Can you work these out from the model? Positions are in its coordinate system, mm. A direction names the side the tool comes from. Round coordinates to 2 decimals unless told otherwise and drop trailing zeros. Loops run counter-clockwise (first coordinate to the right, second up) from the corner with the lowest first, then second, coordinate; pieces in that order, holes last. Notation, with made-up numbers: (-39.75, 86) -> (-32.75, 86) arc R21 ccw to (-32.75, 117) -> close; hole circle Ø5 at (-37.75, 57.25). An arc over 180 degrees is marked (long way). Use a Markdown table: item, result.
Autodesk Inventor part; units mm, degrees
ref_plane "YZ Plane" through (0, 0, 0) normal (1, 0, 0) x (0, 1, 0)
ref_plane "XZ Plane" through (0, 0, 0) normal (0, 1, 0) x (-1, 0, 0)
ref_plane "XY Plane" through (0, 0, 0) normal (0, 0, 1) x (1, 0, 0)
sketch "Sketch1" plane through (0, 0, 0) normal (0, 1, 0) x (-1, 0, 0)
  arc A0 (23.1118, 83.4134) -> (26.1118, 83.4134) centre (24.6118, 83.4134) ccw
  line L0 (23.1118, 98.4134) -> (23.1118, 83.4134)
  arc A1 (26.1118, 98.4134) -> (23.1118, 98.4134) centre (24.6118, 98.4134) ccw
  line L1 (26.1118, 83.4134) -> (26.1118, 98.4134)
  arc A2 (16.2641, 134.7212) -> (19.2641, 134.7212) centre (17.7641, 134.7212) ccw
  line L2 (16.2641, 149.7212) -> (16.2641, 134.7212)
  arc A3 (19.2641, 149.7212) -> (16.2641, 149.7212) centre (17.7641, 149.7212) ccw
  line L3 (19.2641, 134.7212) -> (19.2641, 149.7212)
  arc A4 (-19.2641, 134.7212) -> (-16.2641, 134.7212) centre (-17.7641, 134.7212) ccw
  line L4 (-19.2641, 149.7212) -> (-19.2641, 134.7212)
  arc A5 (-16.2641, 149.7212) -> (-19.2641, 149.7212) centre (-17.7641, 149.7212) ccw
  line L5 (-16.2641, 134.7212) -> (-16.2641, 149.7212)
  arc A6 (-26.1118, 83.4134) -> (-23.1118, 83.4134) centre (-24.6118, 83.4134) ccw
  line L6 (-26.1118, 98.4134) -> (-26.1118, 83.4134)
  arc A7 (-23.1118, 98.4134) -> (-26.1118, 98.4134) centre (-24.6118, 98.4134) ccw
  line L7 (-23.1118, 83.4134) -> (-23.1118, 98.4134)
  circle A8 centre (-24.2029, 34.3759) radius 1.5
  circle A9 centre (-13.2835, 163.8268) radius 1.5
  circle A10 centre (24.2029, 129.4508) radius 1.5
  circle A11 centre (13.2835, 0) radius 1.5
  arc A12 (-31.7205, 55.8278) -> (-31.7205, 107.999) centre (-139.6118, 81.9134) ccw
  arc A13 (-31.7205, 55.8278) -> (-31.2853, 43.4596) centre (-9.3646, 50.4227) ccw
  line L8 (-31.2853, 43.4596) -> (-17.0958, -1.211)
  arc A14 (-17.0958, -1.211) -> (-9.2835, 0) centre (-13.2835, 0) ccw
  arc A15 (9.2835, 0) -> (-9.2835, 0) centre (0, 0) ccw
  arc A16 (9.2835, 0) -> (17.0958, -1.211) centre (13.2835, 0) ccw
  line L9 (17.0958, -1.211) -> (31.2853, 43.4596)
  arc A17 (31.2853, 43.4596) -> (31.7205, 55.8278) centre (9.3646, 50.4227) ccw
  arc A18 (31.7205, 107.999) -> (31.7205, 55.8278) centre (139.6118, 81.9134) ccw
  arc A19 (31.7205, 107.999) -> (31.2853, 120.3671) centre (9.3646, 113.4041) ccw
  line L10 (31.2853, 120.3671) -> (17.0958, 165.0377)
  arc A20 (17.0958, 165.0377) -> (14.6505, 167.5859) centre (13.2835, 163.8268) ccw
  line L11 (14.6505, 167.5859) -> (2.0505, 172.1678)
  arc A21 (2.0505, 172.1678) -> (-2.0505, 172.1678) centre (0, 166.529) ccw
  line L12 (-2.0505, 172.1678) -> (-14.6505, 167.5859)
  arc A22 (-14.6505, 167.5859) -> (-17.0958, 165.0377) centre (-13.2835, 163.8268) ccw
  line L13 (-17.0958, 165.0377) -> (-31.2853, 120.3671)
  arc A23 (-31.2853, 120.3671) -> (-31.7205, 107.999) centre (-9.3646, 113.4041) ccw
  circle A24 centre (24.2029, 34.3759) radius 1.5
  circle A25 centre (13.2835, 163.8268) radius 1.5
  circle A26 centre (-24.2029, 129.4508) radius 1.5
  circle A27 centre (-13.2835, 0) radius 1.5
  point P0 (31.7205, 107.999)
  point P1 (31.2853, 120.3671)
  point P2 (17.0958, 165.0377)
  point P3 (14.6505, 167.5859)
  point P4 (-31.7205, 55.8278)
  point P5 (-31.2853, 43.4596)
  point P6 (-17.0958, -1.211)
  point P7 (-9.2835, 0)
  point P8 (9.2835, 0)
  point P9 (31.7205, 55.8278)
  point P10 (19.2641, 149.7212)
  point P11 (16.2641, 149.7212)
  point P12 (23.1118, 98.4134)
extrude "Extrusion1" add sketch "Sketch1" along normal blind 3
properties part number "399 prig top plate"
1. I want a section at C-C (y = 1.5). State how many separate pieces and enclosed holes the cut face has, plus the area to 3 significant figures.
Answer sheet:
| item | result |
|---|---|
| separate pieces | 1 |
| enclosed holes | 12 |
| area | 8,770 mm² |
2. Which directions (+Z, -Z, +X, -X, +Y, -Y) give clear straight access to the entire face, cutting with the end or side of a thin tool? Please do faces 1 (the flat face through (19.264, 1, 142)), 2 (the flat face through (24.29, 1.48, 21.44)).
Answer sheet:
| item | result |
|---|---|
| face 1 | +Y, -Y |
| face 2 | -Z, +X, +Y, -Y |
3. I want a section at B-B (x = 0). Please give me the cut outline in (y, z).
Answer sheet:
| item | result |
|---|---|
| outline | (0, 9.28) -> (3, 9.28) -> (3, 172.53) -> (0, 172.53) -> close |
4. I want a section at A-A (z = 93.5). Please give me the cut outline in (x, y).
Answer sheet:
| item | result |
|---|---|
| outline | (-29.22, 0) -> (-26.11, 0) -> (-26.11, 3) -> (-29.22, 3) -> close; (-23.11, 0) -> (23.11, 0) -> (23.11, 3) -> (-23.11, 3) -> close; (26.11, 0) -> (29.22, 0) -> (29.22, 3) -> (26.11, 3) -> close |
5. If we mould it in two halves opening along Z, with no side actions, what happens to faces 3 (the cylindrical face through (32.353, 1.479, 114.125)), 4 (the cylindrical face through (12.59, 1.48, -3.94)), 5 (the flat face through (24.09, 1.48, 143.02))? For each: +Z half, -Z half, draft (parallel to the pull), parting line (faces both ways), or undercut.
Answer sheet:
| item | result |
|---|---|
| face 3 | undercut |
| face 4 | -Z half |
| face 5 | +Z half |
6. I need wall thicknesses on line 1 (X direction, y = 2.65, z = 138); line 2 (X direction, y = 1.6, z = 83); line 3 (Z direction, x = -16.5, y = 2.85). Which ranges of each line are inside material? Lowest first, please.
Answer sheet:
| item | result |
|---|---|
| line 1 | x = -25.68 to -19.26, -16.26 to 16.26, 19.26 to 25.68 |
| line 2 | x = -28.62 to -26.05, -23.17 to 23.17, 26.05 to 28.62 |
| line 3 | z = -2.38 to 133.91, 150.53 to 166.2 |
7. I want a section at D-D (z = 155). Please give me the cut outline in (x, y).
Answer sheet:
| item | result |
|---|---|
| outline | (-20.28, 0) -> (20.28, 0) -> (20.28, 3) -> (-20.28, 3) -> close |
8. Will these pins go through, and if not, where does the flat tip stop? pin 1 Ø1 at (y, z) = (2.5, 121.5) entering from +X; pin 2 Ø0.9 at (y, z) = (1.5, 94.5) entering from -X; pin 3 Ø2.5 at (x, z) = (13.28, 0) entering from +Y; pin 4 Ø0.9 at (y, z) = (2, 141.5) entering from +X.
Answer sheet:
| item | result |
|---|---|
| pin 1 | stops at x = 31.08 |
| pin 2 | stops at x = -29.38 |
| pin 3 | passes through |
| pin 4 | stops at x = 24.72 |
